The listing builds one solid part. Answer for the finished solid, in the listing's coordinates (mm). Give positions to 0.01 mm unless a question says otherwise; leave off trailing zeros.
Item 1: The mould has two halves that part along Y. Classify faces 1 (the face through (3, 81.79, 1)), 2 (the face through (3, -81.79, 1)), 3 (the face through (17, -10, 1)): pulls with the +Y half, pulls with the -Y half, needs draft (parallel to the pull), parting line crosses it, or undercut.
Item 2: This flat-tipped pin is pushed along its axis until it touches: pin 1 Ø4 at (x, y) = (2, 58.5) entering from +Z. Where does it stop, or does it pass through?
Item 3: Consider line 1 along Y through (x, z) = (-1, 2); line 2 along Y through (x, z) = (13.5, 1.55); line 3 along X through (y, z) = (-73.5, 0.85). Determine where each line is inside the solid, lowest interval first.
from build123d import *

# Parameters (mm, degrees)
SZKIC1_W                    = 93.394041507
SZKIC1_H                    = 81.79044571
SZKIC1_R                    = 1.5
DODANIE_WYCI_GNI_CIE2_DEPTH = 3


with BuildPart() as part:
    # Szkic1 → Dodanie-wyciągnięcie2 (new body)
    with BuildSketch(Plane.XY):
        with Locations((3.432858123, 40.895222855)):
            Rectangle(SZKIC1_W, SZKIC1_H)
        with Locations((-1, 11)):
            Circle(SZKIC1_R, mode=Mode.SUBTRACT)
        with Locations((18.5, 10)):
            Circle(SZKIC1_R, mode=Mode.SUBTRACT)
        with Locations((-6, 13)):
            Circle(SZKIC1_R, mode=Mode.SUBTRACT)
        with Locations((2, 58.5)):
            Circle(SZKIC1_R, mode=Mode.SUBTRACT)
        with Locations((13.5, 58.5)):
            Circle(SZKIC1_R, mode=Mode.SUBTRACT)
        with Locations((-4, 73.5)):
            Circle(SZKIC1_R, mode=Mode.SUBTRACT)
        with Locations((7.5, 73.5)):
            Circle(SZKIC1_R, mode=Mode.SUBTRACT)
    dodanie_wyci_gni_cie2 = extrude(amount=DODANIE_WYCI_GNI_CIE2_DEPTH)

    # Lustro4: Dodanie-wyciągnięcie2 across plane
    add(dodanie_wyci_gni_cie2.mirror(Plane.ZX))


solid = part.part
Worked answers:
1. face 1: pulls with the +Y half
1. face 2: pulls with the -Y half
1. face 3: undercut
2. pin 1: stops at z = 3
3. line 1: y = -81.79 to -12.5, -9.5 to 9.5, 12.5 to 81.79
3. line 2: y = -81.79 to -60, -57 to 57, 60 to 81.79
3. line 3: x = -43.26 to -5.5, -2.5 to 6, 9 to 50.13
